```python
from build123d import *

# Parameters (mm, degrees)
F1_DEPTH      = 7.493
F1_DEPTH_BACK = 7.493
F3_D          = 5.1054
F4_W          = 7.493
F4_H          = 2.8448
F4_H_2        = 3.302
F5_DEPTH      = 25.4
F8_R          = 1.27
F9_R          = 1.27


with BuildPart() as f1:
    # F0 (on Front) → F1 (new body, two sides)
    with BuildSketch(Plane.XZ) as f1_sk:
        with BuildLine():
            Line((-19.05, -7.493), (19.05, -7.493))
            ThreePointArc((19.05, -7.493), (11.557, 0), (19.05, 7.493))
            Line((19.05, 7.493), (-19.05, 7.493))
            Line((-19.05, 7.493), (-19.05, -7.493))
        make_face()
        with BuildLine():
            ThreePointArc((19.05, 7.493), (11.557, 0), (19.05, -7.493))
            Line((19.05, -7.493), (19.05, 7.493))
        make_face()
        with BuildLine():
            Line((19.05, 7.493), (19.05, -7.493))
            ThreePointArc((19.05, -7.493), (24.3483511114, -5.2983511114), (26.543, 0))
            ThreePointArc((26.543, 0), (24.3483511114, 5.2983511114), (19.05, 7.493))
        make_face()
    extrude(amount=F1_DEPTH)
    extrude(f1_sk.sketch, amount=-F1_DEPTH_BACK)

    # F3 (through all)
    with Locations(Plane.XZ.offset(7.493)):
        with Locations((19.05, 0)):
            Hole(F3_D / 2)

    # F4 (on face) → F5 (cut)
    with BuildSketch(Plane.XY.offset(7.493)):
        with Locations((15.3035, 6.0706)):
            Rectangle(F4_W, F4_H)
        with Locations((22.7965, 6.0706)):
            Rectangle(F4_W, F4_H)
        with Locations((22.7965, 0)):
            Rectangle(F4_W, F4_H_2)
        with Locations((15.3035, 0)):
            Rectangle(F4_W, F4_H_2)
        with Locations((15.3035, -6.0706)):
            Rectangle(F4_W, F4_H)
        with Locations((22.7965, -6.0706)):
            Rectangle(F4_W, F4_H)
    extrude(amount=-F5_DEPTH, mode=Mode.SUBTRACT)

    # F6 (on Front) → F7 (revolve)
    with BuildSketch(Plane.XZ):
        with BuildLine():
            Line((-41.8195042998, 0), (-25.0555042998, 0))
            ThreePointArc((-25.0555042998, 0), (-25.2714088729, 1.8901876837), (-25.908, 3.683))
            ThreePointArc((-25.908, 3.683), (-35.3276919835, 8.1660954268), (-41.8195042998, 0))
        make_face()
        with BuildLine():
            Line((-25.0555042998, 0), (-19.05, 0))
            Line((-19.05, 0), (-19.05, 3.683))
            Line((-19.05, 3.683), (-25.908, 3.683))
            ThreePointArc((-25.908, 3.683), (-25.2714088729, 1.8901876837), (-25.0555042998, 0))
        make_face()
    revolve(axis=Axis((-30.4347521499, 0, 0), (-1, 0, 0)))

    # F8
    f8_edges = [f1.edges().sort_by_distance(p)[0] for p in [
        (-25.908, 0, -3.683),
        (-19.05, 0, -3.683),
    ]]
    fillet(f8_edges, radius=F8_R)

    # F9
    f9_edges = [f1.edges().sort_by_distance(p)[0] for p in [
        (-19.05, -7.493, 0),
        (-19.05, 0, 7.493),
        (-3.7465, -7.493, 7.493),
        (-3.7465, 7.493, 7.493),
        (-19.05, 7.493, 0),
        (-19.05, 0, -7.493),
        (-3.7465, 7.493, -7.493),
        (-3.7465, -7.493, -7.493),
    ]]
    fillet(f9_edges, radius=F9_R)


solid = f1.part
```
Work out the finished part from the listing and answer in its coordinate system (mm). A direction names the side the tool comes from. Give positions to 0.01 mm unless a question says otherwise; leave off trailing zeros. Loops run counter-clockwise (first coordinate to the right, second up) from the corner with the lowest first, then second, coordinate; pieces in that order, holes last. Notation, with made-up numbers: (36, 10.25) -> (55, 10.25) arc R37 ccw to (55, 48.25) -> close; hole circle Ø9 at (36, 51.25). An arc over 180 degrees is marked (long way). Put each result on its own line as item: value. Start each with the question number.
Item 1: The mould has two halves that part along Z. Classify faces 6 (the face through (16.7, -3.1, -1)), 7 (the face through (26.54, -3.17, -0.16)), 8 (the face through (-19.05, -4.2, 2.9)): released by +Z, released by -Z, zero draft, split by the parting line, or undercut.
Item 2: Find the intervals of material crossed by L1, parallel to Z at x = 19.05, y = 3.2; L2, parallel to Y at x = 21.5, z = -2.25; L3, parallel to X at y = -3.5, z = 1.75, in increasing order. Write a range as [from, to].
Item 3: The part is cut by section B-B (z = 0). State how many separate pieces and enclosed holes the cut face has, then the cut area to 3 significant figures.
Item 4: Which of the six approach directions +Z, -Z, +X, -X, +Y, -Y give full straight-line access (tool end or side, diameter ignored) to faces 1 (the face through (16, -4.648, 0)), 2 (the face through (1, 0, 7.493)), 3 (the face through (-18.7, 0.1, -7.1)), 4 (the face through (16, 4.648, 0)), 5 (the face through (-18.7, 0.1, 7.1))?
Item 5: The part is cut by section A-A (x = 3). Give the vertices of the cut face in (y, z).
Item 6: Each of these flat-tipped pins is pushed along its axis until it touches: P1, Ø3, axis at y = -6.5, z = 0, coming from the +X side; P2, Ø3, axis at x = -28, z = 1, coming from the +Y side; P3, Ø4.5, axis at x = 18, z = 0.5, coming from the -Y side; P4, Ø3, axis at x = 19.05, z = 0, coming from the +Y side. Where does it stop, or does it pass through?
Answers below:
1. face 6: undercut
1. face 7: split by the parting line
1. face 8: zero draft
2. L1: [-7.49, -2.55], [2.55, 7.49]
2. L2: [-4.65, -1.65], [1.65, 4.65]
2. L3: [-40.85, -25.88], [-19.59, 17.19], [20.91, 26.34]
3. separate pieces: 3
3. enclosed holes: 0
3. area: 785 mm2
4. face 1: +Z, -Z, +X, -Y
4. face 2: +Z, +X, +Y, -Y
4. face 3: -Z, +Y, -Y
4. face 4: +Z, -Z, +X, +Y
4. face 5: +Z, +Y, -Y
5. outline: (-7.49, -6.22) arc R1.27 ccw to (-6.22, -7.49) -> (6.22, -7.49) arc R1.27 ccw to (7.49, -6.22) -> (7.49, 6.22) arc R1.27 ccw to (6.22, 7.49) -> (-6.22, 7.49) arc R1.27 ccw to (-7.49, 6.22) -> close
6. P1: x = 11.56
6. P2: y = 7.35
6. P3: y = -4.65
6. P4: through
